from build123d import *

# Parameters (mm, degrees)
SKETCH1_W           = 280
SKETCH1_H           = 70
BOSS_EXTRUDE1_DEPTH = 7
FILLET1_R           = 6
SKETCH2_R           = 15
SKETCH2_R_2         = 4
SKETCH2_R_3         = 3
CUT_EXTRUDE1_DEPTH  = 10
BOSS_EXTRUDE2_START = 2
SKETCH3_R           = 20
SKETCH3_R_2         = 15
BOSS_EXTRUDE2_DEPTH = 2
CUT_EXTRUDE2_DEPTH  = 3


with BuildPart() as part:
    # Sketch1 → Boss-Extrude1 (new body)
    with BuildSketch(Plane.XY):
        Rectangle(SKETCH1_W, SKETCH1_H)
    extrude(amount=BOSS_EXTRUDE1_DEPTH)

    # Fillet1
    fillet1_edges = [part.edges().sort_by_distance(p)[0] for p in [
        (140, -35, 3.5),
        (-140, -35, 3.5),
        (-140, 35, 3.5),
        (140, 35, 3.5),
    ]]
    fillet(fillet1_edges, radius=FILLET1_R)

    # Sketch2 → Cut-Extrude1 (cut)
    with BuildSketch(Plane(origin=(0, 0, 0), x_dir=(-1, 0, 0), z_dir=(0, 0, -1))):
        with Locations((-107.5, 0)):
            Circle(SKETCH2_R)
        with Locations((107.5, 0)):
            Circle(SKETCH2_R)
        with Locations((130, 25)):
            Circle(SKETCH2_R_2)
        with Locations((65, 25)):
            Circle(SKETCH2_R_2)
        with Locations((-65, 25)):
            Circle(SKETCH2_R_2)
        with Locations((-130, 25)):
            Circle(SKETCH2_R_2)
        with Locations(Location((-130, -25, 0), (0, 0, 180))):
            Circle(SKETCH2_R_2)
        with Locations(Location((-65, -25, 0), (0, 0, 180))):
            Circle(SKETCH2_R_2)
        with Locations(Location((65, -25, 0), (0, 0, 180))):
            Circle(SKETCH2_R_2)
        with Locations(Location((130, -25, 0), (0, 0, 180))):
            Circle(SKETCH2_R_2)
        with Locations((-132.5, 0)):
            Circle(SKETCH2_R_3)
        with Locations((-107.5, 25)):
            Circle(SKETCH2_R_3)
        with Locations((-107.5, -25)):
            Circle(SKETCH2_R_3)
        with Locations((-82.5, 0)):
            Circle(SKETCH2_R_3)
        with BuildLine():
            Line((2.5, 20.383453672), (2.5, 2.5))
            ThreePointArc((2.5, 2.5), (0, 0), (-2.5, 2.5))
            Line((-2.5, 2.5), (-2.5, 20.383453672))
            ThreePointArc((-2.5, 20.383453672), (0, 30.25), (2.5, 20.383453672))
        make_face()
    extrude(amount=-CUT_EXTRUDE1_DEPTH, mode=Mode.SUBTRACT)

    # Sketch3 → Boss-Extrude2 (add)
    # profile 1 of 2: a face of its own
    with BuildSketch(Plane(origin=(0, 0, 0), x_dir=(-1, 0, 0), z_dir=(0, 0, -1)).offset(BOSS_EXTRUDE2_START)):
        with Locations(Location((-107.5, 0, 0), (0, 0, 180))):
            Circle(SKETCH3_R)
        with Locations((-107.5, 0)):
            Circle(SKETCH3_R_2, mode=Mode.SUBTRACT)
    # profile 2 of 2: a face of its own
    with BuildSketch(Plane(origin=(0, 0, 0), x_dir=(-1, 0, 0), z_dir=(0, 0, -1)).offset(BOSS_EXTRUDE2_START)):
        with Locations(Location((107.5, 0, 0), (0, 0, 180))):
            Circle(SKETCH3_R)
        with Locations((107.5, 0)):
            Circle(SKETCH3_R_2, mode=Mode.SUBTRACT)
    extrude(amount=-BOSS_EXTRUDE2_DEPTH)

    # Sketch4 → Cut-Extrude2 (cut)
    with BuildSketch(Plane.XY.offset(5)):
        with BuildLine():
            Line((-5.25, 20.383453672), (-5.25, 25))
            Line((-5.25, 25), (0, 25))
            Line((0, 25), (5.25, 25))
            Line((5.25, 25), (5.25, 20.383453672))
            Line((5.25, 20.383453672), (5.25, 2.5))
            ThreePointArc((5.25, 2.5), (0, -2.75), (-5.25, 2.5))
            Line((-5.25, 2.5), (-5.25, 20.383453672))
        make_face()
    extrude(amount=-CUT_EXTRUDE2_DEPTH, mode=Mode.SUBTRACT)


solid = part.part
Check sheet for the modelled part. Datum: model origin and axes. Units: mm. A direction names the side the tool comes from. Give positions to 0.01 mm unless a question says otherwise; leave off trailing zeros. Loops run counter-clockwise (first coordinate to the right, second up) from the corner with the lowest first, then second, coordinate; pieces in that order, holes last. Notation, with made-up numbers: M 4,-10.5 L 42,-10.5 A20 ccw 42,-6.5 Z; hole C -6.5,83 d11. An arc over 180 degrees is marked long. Return JSON: item names as keys, results as strings. Group by question number.
1. Cross-section at D-D on y = -7. Record the boundary of the cut face in (x, z) (1 decimal).
2. Mould release check, pull along Y, two halves, no side actions. Record for faces 4 (the cylindrical face through (109.9, -26.8, 3.5)), 5 (the flat face through (110, -15, -2)), 6 (the cylindrical face through (61.185, 26.201, 3.451)), 7 (the cylindrical face through (-127.48, -0.88, -1.01)): released by +Y, released by -Y, zero draft, split by the parting line, or undercut.
3. Cross-section at A-A on x = 0. Record the boundary of the cut face in (y, z), plus the area to 3 significant figures.
4. Cross-section at B-B on z = 3.5. State how many separate pieces and enclosed holes the cut face has, plus the area to 3 significant figures.
5. Go/stop test with flat-tipped pins: pin 1 (9 mm diameter, centred on x = 130, y = 25, fed in from +Z); pin 2 (21 mm diameter, centred on x = 16.5, y = 12, fed in from -Z). Record where each tip stops, or that it passes through.
6. Tool access check on faces 1 (the flat face through (-2, 0, 0)), 2 (the flat face through (-2, 35, 3)), 3 (the flat face through (4, 8, 5)). Record the directions out of +Z, -Z, +X, -X, +Y, -Y that give a thin tool (end or side, any length) a straight path to the whole face; none if there is none.
7. Cross-section at C-C on y = -25. Record the boundary of the cut face in (x, z).
8. Thickness scan on L1, parallel to Y at x = 107.5, z = 4.25; L2, parallel to X at y = 12.5, z = 3; L3, parallel to X at y = -1, z = 0.75. Record the ranges inside material, lowest first.
Return value:
{
 "1": {"outline": "M -140,0 L -126.2,0 L -126.2,-2 L -120.8,-2 L -120.8,7 L -140,7 Z; M -94.2,-2 L -88.8,-2 L -88.8,0 L 88.8,0 L 88.8,-2 L 94.2,-2 L 94.2,7 L -94.2,7 Z; M 120.8,-2 L 126.2,-2 L 126.2,0 L 140,0 L 140,7 L 120.8,7 Z"},
 "2": {"face 4": "undercut", "face 5": "zero draft", "face 6": "undercut", "face 7": "split by the parting line"},
 "3": {"outline": "M -35,0 L 0,0 L 0,2 L -2.75,2 L -2.75,5 L 0,5 L 0,7 L -35,7 Z; M 30.25,0 L 35,0 L 35,7 L 30.25,7 Z", "area": "270 mm^2"},
 "4": {"separate pieces": "1", "enclosed holes": "15", "area": "17,300 mm^2"},
 "5": {"pin 1": "z = 7", "pin 2": "z = 0"},
 "6": {"face 1": "-Z", "face 2": "+Z, -Z, +X, -X, +Y", "face 3": "none"},
 "7": {"outline": "M -140,0 L -134,0 L -134,7 L -140,7 Z; M -126,0 L -69,0 L -69,7 L -126,7 Z; M -61,0 L 61,0 L 61,7 L -61,7 Z; M 69,0 L 104.5,0 L 104.5,7 L 69,7 Z; M 110.5,0 L 126,0 L 126,7 L 110.5,7 Z; M 134,0 L 140,0 L 140,7 L 134,7 Z"},
 "8": {"L1": "-35 to -28, -22 to -15, 15 to 22, 28 to 35", "L2": "-140 to -115.79, -99.21 to -5.25, 5.25 to 99.21, 115.79 to 140", "L3": "-140 to -122.47, -92.53 to 79.67, 85.33 to 92.53, 122.47 to 129.67, 135.33 to 140"}
}
